Work out the finished part from the listing and answer in its coordinate system (mm). Give positions to 0.01 mm unless a question says otherwise; leave off trailing zeros. Write each loop counter-clockwise with the first axis right and the second up, starting at its lowest first coordinate (ties: lowest second). Pieces come first, ordered by that corner, then holes. Notation, with made-up numbers: (83.25, -8.5) -> (109.25, -8.5) arc R19 ccw to (109.25, 17.5) -> close; hole circle Ø7 at (60, 17.5). An arc over 180 degrees is marked (long way). Use a Markdown table: item, result. Add a question column.
Q1. For a pull along X with two mould halves and no side action, classify faces 1 (the face through (-49.172, -15.345, 1.479)), 2 (the face through (-1, 1, 0)), 3 (the face through (-12.05, 54.28, 1.48)) as pulls with the +X half, pulls with the -X half, needs draft (parallel to the pull), parting line crosses it, or undercut.
Q2. Section D-D, the plane y = 44 is taken. Give the vertices of the cut face in (x, z).
Q3. Section C-C, the plane x = -47 is taken. Give the vertices of the cut face in (y, z).
Q4. Consider line 1 (Y direction, x = 47.5, z = 2.85); line 2 (X direction, y = -41, z = 0.3); line 3 (Y direction, x = -49, z = 1.3). Determine where each line is inside the solid, lowest interval first.
Q5. Section A-A, the plane x = 0 is taken. Give the vertices of the cut face in (y, z), plus the area to 3 significant figures.
Q6. Each of these flat-tipped pins is pushed along its axis until it touches: pin 1 Ø3 at (x, y) = (-29.15, 40.13) entering from -Z; pin 2 Ø1.5 at (x, z) = (-43.5, 1.5) entering from -Y. Where does it stop, or does it pass through?
Autodesk Inventor part; units mm, degrees
ref_plane "YZ Plane" through (0, 0, 0) normal (1, 0, 0) x (0, 1, 0)
ref_plane "XZ Plane" through (0, 0, 0) normal (0, 1, 0) x (-1, 0, 0)
ref_plane "XY Plane" through (0, 0, 0) normal (0, 0, 1) x (1, 0, 0)
ref_plane "Work Plane1" through (0, 0, 0) normal (0, 0, 1) x (1, 0, 0)
sketch "Sketch1" plane through (0, 0, 0) normal (0, 0, 1) x (1, 0, 0)
  circle A0 centre (0, 0) radius 55.6
extrude "Extrusion1" add sketch "Sketch1" along normal blind 3
sketch "Sketch2" plane through (0, 0, 3) normal (0, 0, 1) x (1, 0, 0)
  circle A0 centre (-29.1541, 40.1272) radius 1.45
  circle A1 centre (-47.1724, 15.3272) radius 1.45
  circle A2 centre (-47.1724, -15.3272) radius 1.45
  circle A3 centre (-29.1541, -40.1272) radius 1.45
  circle A4 centre (0, -49.6) radius 1.45
  circle A5 centre (29.1541, -40.1272) radius 1.45
  circle A6 centre (47.1724, -15.3272) radius 1.45
  circle A7 centre (47.1724, 15.3272) radius 1.45
  circle A8 centre (29.1541, 40.1272) radius 1.45
  circle A9 centre (0, 49.6) radius 1.45
  circle A10 centre (0, 0) radius 55.6
  circle A11 centre (0, 0) radius 44.6
hole "Hole1" at (0, -49.6, 3) direction (0, 0, -1) diameter 4 end through all
pattern_circular "Circular Pattern1" count 10 over 360 about axis through (0, 0, 0) along (0, 0, 1) of "Hole1"
sketch "Sketch3" plane through (0, 0, 3) normal (0, 0, 1) x (1, 0, 0)
  circle A0 centre (-29.1541, -40.1272) radius 2
  circle A1 centre (-47.1724, -15.3272) radius 2
  circle A2 centre (-47.1724, 15.3272) radius 2
  circle A3 centre (-29.1541, 40.1272) radius 2
  circle A4 centre (0, 49.6) radius 2
  circle A5 centre (29.1541, 40.1272) radius 2
  circle A6 centre (47.1724, 15.3272) radius 2
  circle A7 centre (47.1724, -15.3272) radius 2
  circle A8 centre (29.1541, -40.1272) radius 2
  circle A9 centre (0, -49.6) radius 2
  circle A10 centre (0, 0) radius 55.6
properties part number "Anglerfish_Frontwindow_3inchtube_V0"
Result set:
| question | item | result |
|---|---|---|
| 1 | face 1 | undercut |
| 1 | face 2 | needs draft |
| 1 | face 3 | parting line crosses it |
| 2 | outline | (-33.99, 0) -> (33.99, 0) -> (33.99, 3) -> (-33.99, 3) -> close |
| 3 | outline | (-29.7, 0) -> (-17.32, 0) -> (-17.32, 3) -> (-29.7, 3) -> close; (-13.33, 0) -> (13.33, 0) -> (13.33, 3) -> (-13.33, 3) -> close; (17.32, 0) -> (29.7, 0) -> (29.7, 3) -> (17.32, 3) -> close |
| 4 | line 1 | y = -28.9 to -17.3, -13.35 to 13.35, 17.3 to 28.9 |
| 4 | line 2 | x = -37.55 to -30.95, -27.35 to 27.35, 30.95 to 37.55 |
| 4 | line 3 | y = -26.27 to -16.14, -14.51 to 14.51, 16.14 to 26.27 |
| 5 | outline | (-55.6, 0) -> (-51.6, 0) -> (-51.6, 3) -> (-55.6, 3) -> close; (-47.6, 0) -> (47.6, 0) -> (47.6, 3) -> (-47.6, 3) -> close; (51.6, 0) -> (55.6, 0) -> (55.6, 3) -> (51.6, 3) -> close |
| 5 | area | 310 mm2 |
| 6 | pin 1 | passes through |
| 6 | pin 2 | stops at y = -35.55 |
